The figure shows three views and two pictorial views of one solid part (mm, origin at its lowest corner). Answer the questions. A direction names the side the tool comes from. Give positions to 0.01 mm unless a question says otherwise; leave off trailing zeros. Write each loop counter-clockwise with the first axis right and the second up, starting at its lowest first coordinate (ties: lowest second). Pieces come first, ordered by that corner, then holes. Notation, with made-up numbers: (-37.75, 28) -> (12.25, 28) arc R20 ccw to (12.25, 48) -> close; hole circle Ø10 at (-6, 78). An arc over 180 degrees is marked (long way). Use a Markdown table: item, result.
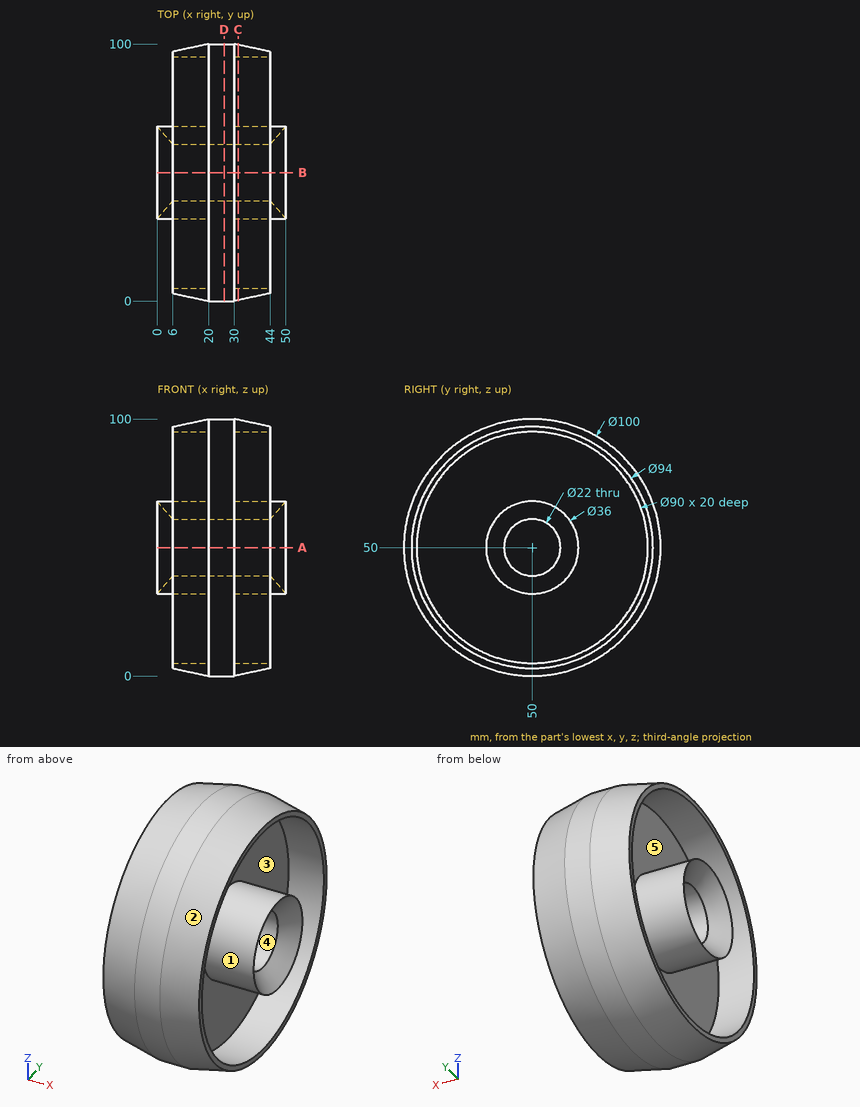
Item 1: For a pull along Z with two mould halves and no side action, classify the marked faces 1 and 2 as +Z half, -Z half, draft (parallel to the pull), parting line (faces both ways), or undercut.
Return value:
| item | result |
|---|---|
| face 1 | undercut |
| face 2 | parting line |
Item 2: A cutting plane is placed at D-D (x = 26). Give the vertices of the cut face in (y, z).
Return value:
| item | result |
|---|---|
| outline | circle Ø100 at (50, 50); hole circle Ø22 at (50, 50) |
Item 3: A cutting plane is placed at A-A (z = 50). Give the vertices of the cut face in (x, y).
Return value:
| item | result |
|---|---|
| outline | (0, 32) -> (20, 32) -> (20, 5) -> (6, 5) -> (6, 3) -> (20, 0) -> (30, 0) -> (44, 3) -> (44, 5) -> (30, 5) -> (30, 32) -> (50, 32) -> (44, 39) -> (6, 39) -> close; (0, 68) -> (6, 61) -> (44, 61) -> (50, 68) -> (30, 68) -> (30, 95) -> (44, 95) -> (44, 97) -> (30, 100) -> (20, 100) -> (6, 97) -> (6, 95) -> (20, 95) -> (20, 68) -> close |
Item 4: A cutting plane is placed at C-C (x = 31.5). Give the vertices of the cut face in (y, z), then the cut area to 3 significant figures.
Return value:
| item | result |
|---|---|
| outline | circle Ø99.36 at (50, 50); circle Ø36 at (50, 50); hole circle Ø90 at (50, 50); hole circle Ø22 at (50, 50) |
| area | 2,030 mm^2 |
Item 5: Each of these flat-tipped pins is pushed along its axis until it touches: P1, Ø4, axis at y = 24.5, z = 36.5, coming from the +X side; P2, Ø3, axis at x = 14.5, z = 55.5, coming from the -Y side; P3, Ø1, axis at y = 26.5, z = 46.5, coming from the -X side. Where does it stop, or does it pass through?
Return value:
| item | result |
|---|---|
| P1 | x = 30 |
| P2 | y = 1.13 |
| P3 | x = 20 |
Item 6: Straight lines are drawn through the part: line 1 along Z through (x, y) = (23, 50); line 2 along Z through (x, y) = (18, 50); line 3 along Y through (x, z) = (38, 59). For each, find the intervals that lie inside material, in ascending order. Write a range as [from, to].
Return value:
| item | result |
|---|---|
| line 1 | [0, 39], [61, 100] |
| line 2 | [0.43, 5], [32, 39], [61, 68], [95, 99.57] |
| line 3 | [2.56, 5.91], [34.41, 43.68], [56.32, 65.59], [94.09, 97.44] |
Item 7: A tool of negligible diameter and unlimited length cuts with its end or side. For the marked faces 3, 4 and 5, from which of +Z, -Z, +X, -X, +Y, -Y can it reach the whole face along a straight path? Write none if from no direction.
Return value:
| item | result |
|---|---|
| face 3 | +X |
| face 4 | +X, -X |
| face 5 | -X |
